```python
from build123d import *

# Parameters (mm, degrees)
F0_W     = 30
F0_H     = 30
F1_DEPTH = 150
F2_R     = 5.25
F3_DEPTH = 30.001
F4_R     = 5.25
F4_R_2   = 3.0375
F5_DEPTH = 30.001
F6_R     = 8.75
F7_DEPTH = 11
F8_R     = 3.0375
F9_DEPTH = 30.001


with BuildPart() as f1:
    # F0 (on Front) → F1 (new body)
    with BuildSketch(Plane.XZ):
        Rectangle(F0_W, F0_H)
    extrude(amount=F1_DEPTH)

    # F2 (on face) → F3 (cut, through all)
    with BuildSketch(Plane(origin=(-15, 0, 0), x_dir=(0, -1, 0), z_dir=(-1, 0, 0))):
        with Locations((8, 0)):
            Circle(F2_R)
        with Locations((75, 0)):
            Circle(F2_R)
        with Locations((142, 0)):
            Circle(F2_R)
    extrude(amount=-F3_DEPTH, mode=Mode.SUBTRACT)

    # F4 (on face) → F5 (cut, through all)
    with BuildSketch(Plane.XY.offset(15)):
        with Locations((0, -37.5)):
            Circle(F4_R)
        with Locations((10, -50)):
            Circle(F4_R_2)
        with Locations((0, -112.5)):
            Circle(F4_R)
        with Locations((10, -100)):
            Circle(F4_R_2)
        with Locations((-10, -50)):
            Circle(F4_R_2)
        with Locations((-10, -100)):
            Circle(F4_R_2)
    extrude(amount=-F5_DEPTH, mode=Mode.SUBTRACT)

    # F6 (on face) → F7 (cut)
    with BuildSketch(Plane.XY.offset(15)):
        with Locations((0, -37.5)):
            Circle(F6_R)
        with Locations((0, -112.5)):
            Circle(F6_R)
    extrude(amount=-F7_DEPTH, mode=Mode.SUBTRACT)

    # F8 (on face) → F9 (cut, through all)
    with BuildSketch(Plane(origin=(-15, 0, 0), x_dir=(0, -1, 0), z_dir=(-1, 0, 0))):
        with Locations((20, 0)):
            Circle(F8_R)
        with Locations((130, 0)):
            Circle(F8_R)
    extrude(amount=-F9_DEPTH, mode=Mode.SUBTRACT)


solid = f1.part
```
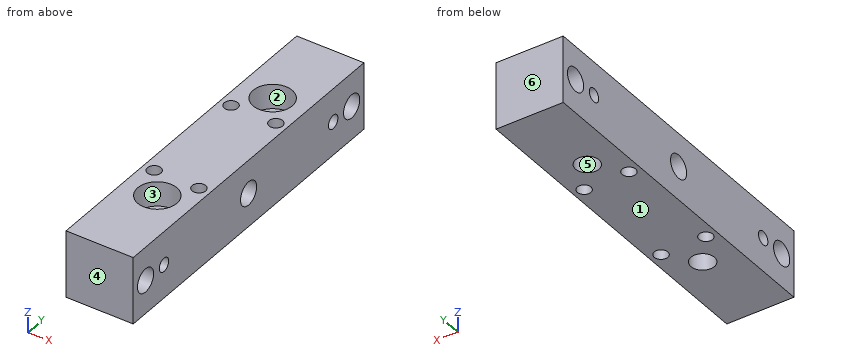
For this review, take the finished solid that the model builds, in its own axes (mm). Face numbers are marked on the shaded views. A direction names the side the tool comes from. Round coordinates to 2 decimals unless told otherwise and drop trailing zeros. Write each loop counter-clockwise with the first axis right and the second up, starting at its lowest first coordinate (ties: lowest second). Pieces come first, ordered by that corner, then holes. Notation, with made-up numbers: (77.5, 60.25) - (117.5, 60.25) arc R21 ccw to (117.5, 81.25) - close; hole circle Ø4 at (-32.5, 79). An arc over 180 degrees is marked (long way). Put each result on its own line as item: value.
Q1. Insertion check: pin 1 Ø3 at (x, y) = (3.5, -115.5) entering from +Z; pin 2 Ø3.5 at (x, y) = (-10, -50) entering from -Z. Each pin has a flat end and moves straight along its axis. Give the tip position at first contact, or say it passes through.
Solved:
pin 1: stops at z = 4
pin 2: passes through
Q2. We need section B-B (y = -50). Give the boundary of the cut face in (x, z), and give its area (4 significant figures).
Solved:
outline: (-15, -15) - (-13.04, -15) - (-13.04, 15) - (-15, 15) - close; (-6.96, -15) - (6.96, -15) - (6.96, 15) - (-6.96, 15) - close; (13.04, -15) - (15, -15) - (15, 15) - (13.04, 15) - close
area: 535.5 mm2
Q3. Machinability: for the marked faces 1 and 2, which of the approach directions +Z, -Z, +X, -X, +Y, -Y give a long, thin tool a straight path to every point of the face, cutting with its end or side? Answer none if there is none.
Solved:
face 1: -Z, +X, -X, +Y, -Y
face 2: +Z
Q4. Wall thickness on probe 1 along Y at (x, z) = (0, 12.75); probe 2 along Y at (x, z) = (4.5, 11.5); probe 3 along Z at (x, y) = (-8, -8): over which ranges is each line inside the solid? List them lowest first.
Solved:
probe 1: y = -150 to -121.25, -103.75 to -46.25, -28.75 to 0
probe 2: y = -150 to -120, -105 to -45, -30 to 0
probe 3: z = -15 to -5.25, 5.25 to 15
Q5. We need section C-C (y = -142). Give the boundary of the cut face in (x, z).
Solved:
outline: (-15, -15) - (15, -15) - (15, -5.25) - (-15, -5.25) - close; (-15, 5.25) - (15, 5.25) - (15, 15) - (-15, 15) - close
Q6. We need section A-A (x = 10). Count the separate pieces of the cut face and the enclosed holes in it, and give its area (3 significant figures).
Solved:
separate pieces: 3
enclosed holes: 5
area: 3,820 mm2
Q7. Mouldability with a two-part tool opening along Y and no side actions: class the marked faces 3, 4, 5 and 6 as released by +Y, released by -Y, zero draft, split by the parting line, or undercut.
Solved:
face 3: undercut
face 4: released by -Y
face 5: undercut
face 6: released by +Y
